from build123d import *

# Parameters (mm, degrees)
BOSS_EXTRU_1_DEPTH      = 10
ESQUISSE2_R             = 2.75
ENL_V_MAT_EXTRU_1_DEPTH = 10
ESQUISSE3_R             = 2.75
ENL_V_MAT_EXTRU_2_DEPTH = 10
ESQUISSE4_R             = 2.75
ENL_V_MAT_EXTRU_3_DEPTH = 10
BOSS_EXTRU_4_DEPTH      = 20


with BuildPart() as part:
    # Esquisse1 → Boss.-Extru.1 (new body, symmetric)
    with BuildSketch(Plane.XY):
        with BuildLine():
            ThreePointArc((-3.184001831, 23.485147058), (0, 23.7), (3.184001831, 23.485147058))
            Line((3.184001831, 23.485147058), (21.930734879, -8.985147058))
            ThreePointArc((21.930734879, -8.985147058), (20.52480207, -11.85), (18.746733049, -14.5))
            Line((18.746733049, -14.5), (-18.746733049, -14.5))
            ThreePointArc((-18.746733049, -14.5), (-20.52480207, -11.85), (-21.930734879, -8.985147058))
            Line((-21.930734879, -8.985147058), (-3.184001831, 23.485147058))
        make_face()
        with BuildLine():
            ThreePointArc((17.738094599, -12.5), (18.792751262, -10.85), (19.694364847, -9.111640537))
            Line((19.694364847, -9.111640537), (1.956270248, 21.611640537))
            ThreePointArc((1.956270248, 21.611640537), (0, 21.7), (-1.956270248, 21.611640537))
            Line((-1.956270248, 21.611640537), (-19.694364847, -9.111640537))
            ThreePointArc((-19.694364847, -9.111640537), (-18.792751262, -10.85), (-17.738094599, -12.5))
            Line((-17.738094599, -12.5), (17.738094599, -12.5))
        make_face(mode=Mode.SUBTRACT)
    extrude(amount=BOSS_EXTRU_1_DEPTH, both=True)

    # Esquisse2 → Enlèv. mat.-Extru.1 (cut, symmetric)
    with BuildSketch(Plane(origin=(20.338733964, -11.742573529, 0), x_dir=(0, 0, 1), z_dir=(-0.866025404, 0.5, 0))):
        Circle(ESQUISSE2_R)
    extrude(amount=ENL_V_MAT_EXTRU_1_DEPTH, both=True, mode=Mode.SUBTRACT)

    # Esquisse3 → Enlèv. mat.-Extru.2 (cut, symmetric)
    with BuildSketch(Plane(origin=(-20.338733964, -11.742573529, 0), x_dir=(0, 0, 1), z_dir=(-0.866025404, -0.5, 0))):
        Circle(ESQUISSE3_R)
    extrude(amount=ENL_V_MAT_EXTRU_2_DEPTH, both=True, mode=Mode.SUBTRACT)

    # Esquisse4 → Enlèv. mat.-Extru.3 (cut, symmetric)
    with BuildSketch(Plane(origin=(0, 23.485147058, 0), x_dir=(-1, 0, 0), z_dir=(0, -1, 0))):
        Circle(ESQUISSE4_R)
    extrude(amount=ENL_V_MAT_EXTRU_3_DEPTH, both=True, mode=Mode.SUBTRACT)

    # Esquisse6 → Boss.-Extru.4 (add)
    with BuildSketch(Plane(origin=(0, 0, -10), x_dir=(-1, 0, 0), z_dir=(0, 0, -1))):
        Polygon((4.907477288, 20.5), (5.907477288, 22.232050808), (10.237604307, 19.732050808), (7.794228634, 15.5), align=None)
    extrude(amount=-BOSS_EXTRU_4_DEPTH)


solid = part.part
Work out the finished part from the listing and answer in its coordinate system (mm). A direction names the side the tool comes from. Round coordinates to 2 decimals unless told otherwise and drop trailing zeros. Loops run counter-clockwise (first coordinate to the right, second up) from the corner with the lowest first, then second, coordinate; pieces in that order, holes last. Notation, with made-up numbers: (38.25, 70) - (43.25, 70) arc R26 cw to (43.25, 107) - close; hole circle Ø10 at (36, 81). An arc over 180 degrees is marked (long way). One line per item, written item: value.
Q1. Find section B-B on x = 0. Give the vertices of the cut face in (y, z).
Check values:
outline: (-14.5, -10) - (-12.5, -10) - (-12.5, 10) - (-14.5, 10) - close; (21.7, -10) - (23.7, -10) - (23.7, -2.75) - (21.7, -2.75) - close; (21.7, 2.75) - (23.7, 2.75) - (23.7, 10) - (21.7, 10) - close
Q2. Find section D-D on z = 1.25. Give the vertices of the cut face in (x, y), and give its area (3 significant figures).
Check values:
outline: (-21.93, -8.99) arc R23.7 ccw to (-21.64, -9.67) - (-19.2, -8.26) - (-2.45, 20.76) - (-2.45, 23.57) arc R23.7 ccw to (-3.18, 23.49) - (-4.91, 20.5) - (-5.91, 22.23) - (-10.24, 19.73) - (-7.79, 15.5) - close; (-19.19, -13.91) arc R23.7 ccw to (-18.75, -14.5) - (18.75, -14.5) arc R23.7 ccw to (19.19, -13.91) - (16.75, -12.5) - (-16.75, -12.5) - close; (2.45, 20.76) - (19.2, -8.26) - (21.64, -9.67) arc R23.7 ccw to (21.93, -8.99) - (3.18, 23.49) arc R23.7 ccw to (2.45, 23.57) - close
area: 236 mm2
Q3. The mould has two halves that part along X. Classify faces 4 (the flat face through (-10, 9, 10)), 5 (the flat face through (-9.033, 17.646, -0.14)), 6 (the cylindrical face through (-18.806, -10.826, -5.91)): +X half, -X half, draft (parallel to the pull), parting line (faces both ways), or undercut.
Check values:
face 4: draft
face 5: -X half
face 6: undercut
Q4. For faces 1 (the flat face through (0, -14.5, 0)), 2 (the cylindrical face through (0, 21.7, 6)), 3 (the cylindrical face through (-2.62, 22.33, -0.83)), determine the directions among +Z, -Z, +X, -X, +Y, -Y from which every point of the face is accessible in a straight line to the end or side of a thin tool.
Check values:
face 1: +Z, -Z, +X, -X, -Y
face 2: +Z, -Z
face 3: +Y
Q5. Find section A-A on z = -5.5. Give the vertices of the cut face in (x, y), and give its area (3 significant figures).
Check values:
outline: (-21.93, -8.99) arc R23.7 ccw to (-18.75, -14.5) - (18.75, -14.5) arc R23.7 ccw to (21.93, -8.99) - (3.18, 23.49) arc R23.7 ccw to (-3.18, 23.49) - (-4.91, 20.5) - (-5.91, 22.23) - (-10.24, 19.73) - (-7.79, 15.5) - close; hole (-19.69, -9.11) arc R21.7 ccw to (-17.74, -12.5) - (17.74, -12.5) arc R21.7 ccw to (19.69, -9.11) - (1.96, 21.61) arc R21.7 ccw to (-1.96, 21.61) - close
area: 267 mm2
Q6. Straight lines are drawn through the part: probe 1 along Z at (x, y) = (0, 22); probe 2 along X at (y, z) = (21.35, 0); probe 3 along X at (y, z) = (21.8, 0). For each, find the intervals that lie inside material, in ascending order.
Check values:
probe 1: -10 to -2.75, 2.75 to 10
probe 2: -7.44 to -5.4, -4.42 to -2.75, 2.75 to 4.42
probe 3: -6.66 to -5.66, -4.16 to -2.75, 2.75 to 4.16
Q7. Each of these flat-tipped pins is pushed along its axis until it touches: pin 1 Ø10 at (y, z) = (8, 1.5) entering from -X; pin 2 Ø5 at (y, z) = (14, -5) entering from +X; pin 3 Ø3 at (y, z) = (1.5, -8) entering from +X. Where does it stop, or does it pass through?
Check values:
pin 1: x = -15.01
pin 2: x = 10.1
pin 3: x = 16.74
Q8. Find section C-C on y = 9. Give the vertices of the cut face in (x, z), and give its area (3 significant figures).
Check values:
outline: (-11.55, -10) - (-9.24, -10) - (-9.24, 10) - (-11.55, 10) - close; (9.24, -10) - (11.55, -10) - (11.55, 10) - (9.24, 10) - close
area: 92.4 mm2
